Work out the finished part from the listing and answer in its coordinate system (mm). A direction names the side the tool comes from. Coordinates: 2 decimals unless noted, no trailing zeros. Write each loop counter-clockwise with the first axis right and the second up, starting at its lowest first coordinate (ties: lowest second). Pieces come first, ordered by that corner, then holes. Notation, with made-up numbers: (-19, -30.75) - (40, -30.75) arc R35 ccw to (40, 7.25) - close; hole circle Ø10 at (-34, -13.5). An arc over 180 degrees is marked (long way). Use a Markdown table: item, result. Add a question column.
(1) The part is cut by section C-C, the plane z = 32.5. Give the vertices of the cut face in (x, y).
(2) Given pin 1 Ø2 at (x, y) = (38, 2) entering from +Z; pin 2 Ø1.9 at (x, y) = (4, 3.5) entering from -Z, each flat-ended and moving along its own axis, determine where each tip first touches the part or whether it passes through.
(3) For a pull along X with two mould halves and no side action, classify faces 4 (the face through (36, 3, -0.015)), 5 (the face through (42.644, 3.131, 50.403)), 6 (the face through (12.318, 3.131, 0.362)) as released by +X, released by -X, zero draft, split by the parting line, or undercut.
(4) Find the intervals of material crossed by line 1 (X direction, y = 6.25, z = 28.5); line 2 (X direction, y = 3.25, z = 27.5); line 3 (Z direction, x = 6, y = 5), in increasing order. Write a range as from..to.
(5) The part is cut by section B-B, the plane z = 4. Give the vertices of the cut face in (x, y).
(6) The part is cut by section D-D, the plane x = 27. Give the vertices of the cut face in (y, z), then the cut area to 3 significant figures.
(7) The part is cut by section A-A, the plane y = 5.25. Give the vertices of the cut face in (x, z) (1 decimal).
(8) A tool of negligible diameter and unlimited length cuts with its end or side. For faces 1 (the face through (21.44, 3.13, 15.34)), 2 (the face through (0.362, 3.131, 0.382)), 3 (the face through (30.306, 3, 35)), from which of +Z, -Z, +X, -X, +Y, -Y can it reach the whole face along a straight path? Write none if from no direction.
Autodesk Fusion 360 part; units mm, degrees
sketch "Sketch1" plane through (0, 0, 0) normal (0, 1, 0) x (1, 0, 0)
  line L0 (0, -1.27) -> (0, -49.53)
  line L1 (1.27, -50.8) -> (11.9668, -50.8)
  line L2 (13.0666, -50.165) -> (30.3061, -20.3053)
  line L3 (30.3061, -20.3053) -> (30.3061, -49.5153)
  line L4 (31.5761, -50.7853) -> (41.7361, -50.7853)
  line L5 (43.0061, -49.5153) -> (43.0061, -1.2553)
  line L6 (41.7361, 0.0147) -> (31.0393, 0.0147)
  line L7 (29.9395, -0.6203) -> (12.7, -30.48)
  line L8 (12.7, -30.48) -> (12.7, -1.27)
  line L9 (11.43, 0) -> (1.27, 0)
  arc A0 (0, -49.53) -> (1.27, -50.8) centre (1.27, -49.53) ccw
  arc A1 (1.27, 0) -> (0, -1.27) centre (1.27, -1.27) ccw
  arc A2 (12.7, -1.27) -> (11.43, 0) centre (11.43, -1.27) ccw
  arc A3 (11.9668, -50.8) -> (13.0666, -50.165) centre (11.9668, -49.53) ccw
  arc A4 (30.3061, -49.5153) -> (31.5761, -50.7853) centre (31.5761, -49.5153) ccw
  arc A5 (41.7361, -50.7853) -> (43.0061, -49.5153) centre (41.7361, -49.5153) ccw
  arc A6 (43.0061, -1.2553) -> (41.7361, 0.0147) centre (41.7361, -1.2553) ccw
  arc A7 (31.0393, 0.0147) -> (29.9395, -0.6203) centre (31.0393, -1.2553) ccw
  point P0 (0, -50.8)
  point P1 (12.7, -50.8)
  point P2 (30.3061, -50.7853)
  point P3 (43.0061, -50.7853)
  point P4 (43.0061, 0.0147)
  point P5 (30.3061, 0.0147)
  point P6 (12.7, 0)
  dimension "d6" = 12.7
  dimension "d7" = 12.7
  dimension "d8" = 12.7
  dimension "d9" = 12.7
  dimension "d11" = 30
  dimension "d12" = 30
  dimension "d13" = 50.8
  dimension "d14" = 50.8
  dimension "d15" = 1.27
  dimension "d16" = 1.27
  dimension "d19" = 43.0061
extrude "Extrude1" add sketch "Sketch1" along normal blind 6.35
Model answer:
| question | item | result |
|---|---|---|
| 1 | outline | (0, 0) - (23.27, 0) - (23.27, 6.35) - (0, 6.35) - close; (30.31, 0) - (43.01, 0) - (43.01, 6.35) - (30.31, 6.35) - close |
| 2 | pin 1 | z = 50.79 |
| 2 | pin 2 | z = 0 |
| 3 | face 4 | zero draft |
| 3 | face 5 | released by +X |
| 3 | face 6 | undercut |
| 4 | line 1 | 0..12.7, 13.84..25.57, 30.31..43.01 |
| 4 | line 2 | 0..12.7, 14.42..26.15, 30.31..43.01 |
| 4 | line 3 | 0..50.8 |
| 5 | outline | (0, 0) - (12.7, 0) - (12.7, 6.35) - (0, 6.35) - close; (27.99, 0) - (43.01, 0) - (43.01, 6.35) - (27.99, 6.35) - close |
| 6 | outline | (0, 5.71) - (6.35, 5.71) - (6.35, 26.03) - (0, 26.03) - close |
| 6 | area | 129 mm^2 |
| 7 | outline | (0, 1.3) arc R1.3 ccw to (1.3, 0) - (11.4, 0) arc R1.3 ccw to (12.7, 1.3) - (12.7, 30.5) - (29.9, 0.6) arc R1.3 ccw to (31, 0) - (41.7, 0) arc R1.3 ccw to (43, 1.3) - (43, 49.5) arc R1.3 ccw to (41.7, 50.8) - (31.6, 50.8) arc R1.3 ccw to (30.3, 49.5) - (30.3, 20.3) - (13.1, 50.2) arc R1.3 ccw to (12, 50.8) - (1.3, 50.8) arc R1.3 ccw to (0, 49.5) - close |
| 8 | face 1 | -Z, +Y, -Y |
| 8 | face 2 | -Z, -X, +Y, -Y |
| 8 | face 3 | +Z, +Y, -Y |
